The drawing under review shows one solid part. Ordinate dimensions are in mm from its lowest x, y, z. A direction names the side the tool comes from. Give positions to 0.01 mm unless a question says otherwise; leave off trailing zeros. Loops run counter-clockwise (first coordinate to the right, second up) from the corner with the lowest first, then second, coordinate; pieces in that order, holes last. Notation, with made-up numbers: (6.5, 5.5) - (16.5, 5.5) arc R10 ccw to (16.5, 23.5) - close; hole circle Ø4 at (-24, 41). An arc over 180 degrees is marked (long way). Write each question's results on one line, items separated by ' | '.
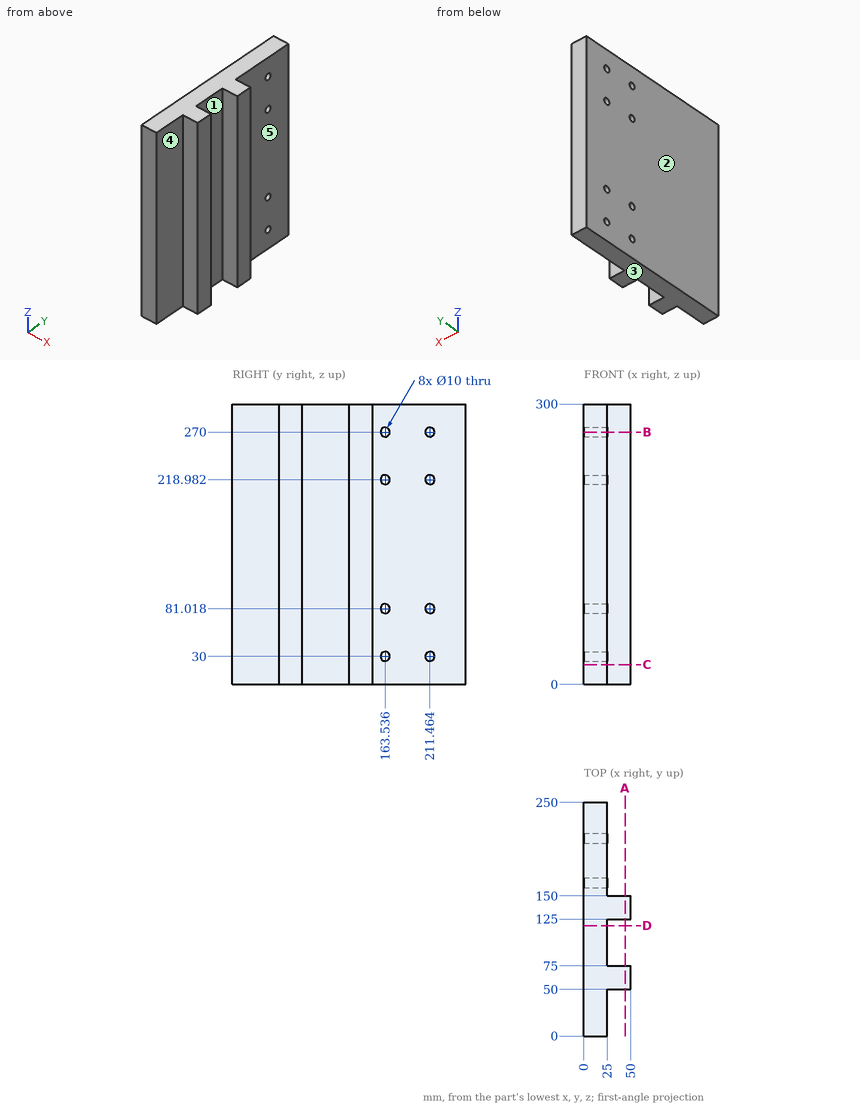
(1) Wall thickness on line 1 along Y through (x, z) = (18, 270) (1 decimal); line 2 along Y through (x, z) = (47.5, 209); line 3 along X through (y, z) = (232, 216): over which ranges is each line inside the solid? List them lowest first. Write a range as from..to.
Answers below:
line 1: 0..158.5, 168.5..206.5, 216.5..250 | line 2: 50..75, 125..150 | line 3: 0..25
(2) Tool access review of the marked faces 1, 2, 3, 4 and 5: name each direction out of +Z, -Z, +X, -X, +Y, -Y from which nothing blocks a thin tool from reaching the whole face with its end or side.
Answers below:
face 1: +Z, -Z, +X | face 2: +Z, -Z, -X, +Y, -Y | face 3: -Z, +X, -X, +Y, -Y | face 4: +Z, -Z, +X, -Y | face 5: +Z, -Z, +X, +Y
(3) Take a section at C-C on z = 21. Give the boundary of the cut face in (x, y).
Answers below:
outline: (0, 0) - (25, 0) - (25, 50) - (50, 50) - (50, 75) - (25, 75) - (25, 125) - (50, 125) - (50, 150) - (25, 150) - (25, 250) - (0, 250) - close
(4) Take a section at A-A on x = 44. Give the boundary of the cut face in (y, z).
Answers below:
outline: (50, 0) - (75, 0) - (75, 300) - (50, 300) - close; (125, 0) - (150, 0) - (150, 300) - (125, 300) - close
(5) Take a section at B-B on z = 270. Give the boundary of the cut face in (x, y) (1 decimal), plus the area to 3 significant figures.
Answers below:
outline: (0, 0) - (25, 0) - (25, 50) - (50, 50) - (50, 75) - (25, 75) - (25, 125) - (50, 125) - (50, 150) - (25, 150) - (25, 158.5) - (0, 158.5) - close; (0, 168.5) - (25, 168.5) - (25, 206.5) - (0, 206.5) - close; (0, 216.5) - (25, 216.5) - (25, 250) - (0, 250) - close | area: 7,000 mm2
(6) Take a section at D-D on y = 118. Give the boundary of the cut face in (x, z).
Answers below:
outline: (0, 0) - (25, 0) - (25, 300) - (0, 300) - close
(7) Insertion check: P1, Ø7.5, axis at x = 36.5, z = 149.5, coming from the +Y side; P2, Ø7.5, axis at x = 35, z = 218.5, coming from the -Y side; P3, Ø25, axis at y = 103.5, z = 186.5, coming from the +X side. Each pin has a flat end and moves straight along its axis. Give the tip position at first contact, or say it passes through.
Answers below:
P1: y = 150 | P2: y = 50 | P3: x = 25
